Autodesk Inventor part; units mm, degrees
ref_plane "Arbeitsebene1" through (0, 0, -100) normal (0, 0, -1) x (-1, 0, 0)
ref_plane "Arbeitsebene3" through (0, 0, -113.5) normal (0, 0, -1) x (-1, 0, 0)
ref_plane "Arbeitsebene4" through (-9.5, -5.25, -113.5) normal (-1, 0, 0) x (0, 0, 1)
sketch "Skizze1" plane through (0, 0, 0) normal (0, 0, 1) x (1, 0, 0)
  line L0 (-9.5, -10.5) -> (7.5, -10.5)
  line L1 (7.5, -10.5) -> (7.5, 10.5)
  line L2 (7.5, 10.5) -> (-9.5, 10.5)
  line L3 (-14.1, 0) -> (18.1, 0)
  line L4 (0, -21.7) -> (0, 21.7)
  line L5 (-9.5, -10.5) -> (-9.5, -15.5)
  line L6 (-9.5, -15.5) -> (13.5, -15.5)
  line L7 (-9.5, 10.5) -> (-9.5, 15.5)
  line L8 (-9.5, 15.5) -> (13.5, 15.5)
  line L9 (13.5, 15.5) -> (13.5, -15.5)
  point P0 (0, 0)
  dimension "d2" = 21
  dimension "d4" = 7.5
  dimension "d5" = 5
  dimension "d8" = 5
  dimension "d9" = 23
  dimension "d147" = 6
  dimension "d148" = 23
extrude "Tower" add sketch "Skizze1" against normal blind 100 contours L0 L4 L6 L5 | L0 L1 L3 L9 L6 L4 | L1 L2 L4 L8 L9 L3 | L2 L7 L8 L4
ref_plane "Arbeitsebene1" through (0, 0, -100) normal (0, 0, -1) x (-1, 0, 0)
sketch "Skizze6" plane through (-9.5, 15.5, 0) normal (0, 1, 0) x (1, 0, 0)
  line L0 (0, 0) -> (23, 0)
  line L1 (0, 0) -> (0, -10)
  line L2 (0, -10) -> (228, -10)
  line L3 (23, 0) -> (23, 100)
  line L4 (0, -10) -> (246, -10)
  line L5 (246, -10) -> (246, 46)
  line L6 (246, 46) -> (224, 46)
  line L7 (246, 46) -> (268, 46) construction
  line L8 (23, 71.167) -> (23, 0)
  line L9 (0, 0) -> (17, 0)
  line L10 (0, 0) -> (0, -12)
  line L11 (246, -12) -> (246, -10)
  spline S0 degree 4 poles (224, 46) (217.2503, 45.4128) (195.5245, 22.479) (125.572, 22.5752) (22.0276, 45.7385) (23, 71.167) knots 0 0 0 0 0 0.374897 1 1 1 1 1
  line L12 (221.3219, 44.8948) -> (192.3718, 31.261) construction
  arc A0 (195.0075, 33.4464) -> (217.9584, 44.255) centre (166.5411, 123.6635) ccw construction
  line L13 (148.8192, 27.3272) -> (94.421, 32.9509) construction
  arc A1 (99.9704, 33.0497) -> (143.4073, 28.5591) centre (158.3015, 384.9585) ccw construction
  line L14 (0, 0) -> (0, 100)
  point P0 (9.5, 0)
  point P1 (206.8469, 38.0779)
  point P2 (121.6201, 30.1391)
  point P3 (23, 70.1618)
  dimension "d34" = 10
  dimension "d38" = 246
  dimension "d39" = 56
  dimension "d40" = 180
  dimension "d41" = 22
extrude "Gripperbogen" add sketch "Skizze6" against normal blind 31 contours L0 L3 S0 L6 L5 L4 L2 L1
sketch "Skizze9" plane through (-9.5, 15.5, 10) normal (0, 0, 1) x (1, 0, 0)
  line L0 (216, -15.5) -> (246, -15.5)
  line L1 (246, 0) -> (246, -31)
  line L2 (216, -15.5) -> (246, -15.5) construction
  line L3 (246, -15.5) -> (246, -31)
  line L4 (224, 0) -> (224, -31)
  line L5 (246, -9.5) -> (224, -9.5)
  line L6 (224, -9.5) -> (224, -6)
  line L7 (224, -6) -> (246, -6)
  line L8 (246, -6) -> (246, -9.5)
  line L9 (0, 0) -> (246, 0)
  line L10 (0, 0) -> (246, 0)
  line L11 (0, 0) -> (0, -31)
  line L12 (246, -31) -> (0, -31)
  line L13 (246, 0) -> (246, -31)
  line L14 (216, -15.5) -> (146, -31)
  point P0 (9.5, -15.5)
  point P1 (246, -6)
  point P2 (235, -6)
  dimension "d61" = 3.5
  dimension "d150" = 6
  dimension "d151" = 6
  dimension "d152" = 100
  dimension "d153" = 30
extrude "Extrusion8" cut sketch "Skizze9" against normal blind 74.5 contours L0 L4 L12 L14 | L0 L1 L12 L4 | L4 L7 L1 L5
sketch "Skizze10" plane through (-9.5, 15.5, -100) normal (0, 1, 0) x (1, 0, 0)
  line L0 (225.7282, -61.6) -> (255.0049, -61.6)
  line L1 (255.0049, -61.6) -> (255.0049, -102.4)
  line L2 (255.0049, -102.4) -> (225.7282, -102.4)
  line L3 (225.7282, -102.4) -> (225.7282, -61.6)
  line L4 (0, -110) -> (246, -110)
  line L5 (246, -54) -> (224, -54)
  point P0 (9.5, -100)
  dimension "d64" = 7.6
  dimension "d65" = 7.6
extrude "Extrusion9" cut sketch "Skizze10" against normal blind 74.5
sketch "Skizze12" plane through (0, 0, -100) normal (0, 0, -1) x (-1, 0, 0)
  line L0 (-214.5, 9.5) -> (-236.5, 9.5)
  line L1 (-236.5, 15.5) -> (-236.5, 9.5)
  line L2 (9.5, 15.5) -> (-236.5, 15.5)
  line L3 (9.5, 15.5) -> (9.5, -15.5)
  line L4 (-136.5, -15.5) -> (9.5, -15.5)
  line L5 (-136.5, -15.5) -> (-206.5, 0)
  line L6 (-206.5, 0) -> (-236.5, 0)
  line L7 (-236.5, 6) -> (-236.5, 0)
  line L8 (-236.5, 6) -> (-214.5, 6)
  line L9 (-214.5, 6) -> (-214.5, 9.5)
  line L10 (-7.5, 10.5) -> (9.5, 10.5)
  line L11 (9.5, 10.5) -> (9.5, 15.5)
  line L12 (9.5, 15.5) -> (-13.5, 15.5)
  line L13 (-13.5, 15.5) -> (-13.5, -15.5)
  line L14 (-13.5, -15.5) -> (9.5, -15.5)
  line L15 (9.5, -15.5) -> (9.5, -10.5)
  line L16 (9.5, -10.5) -> (-7.5, -10.5)
  line L17 (-7.5, -10.5) -> (-7.5, 10.5)
  line L18 (-13.5, 15.5) -> (-13.5, -15.5)
  line L19 (-13.5, -15.5) -> (9.5, -15.5)
  line L20 (9.5, -15.5) -> (9.5, 15.5)
  line L21 (9.5, 15.5) -> (-13.5, 15.5)
  line L22 (-13.5, 15.5) -> (-13.5, -15.5)
  point P0 (9.5, 25.25)
  point P1 (-13.5, -5.25)
  point P2 (-13.5, 15.5)
extrude "Extrusion10" add sketch "Skizze12" against normal blind 10 contours L2 L3 L10 L17 L16 L4 L13 | L3 L16 L17 L10
ref_plane "Arbeitsebene3" through (0, 0, -113.5) normal (0, 0, -1) x (-1, 0, 0)
ref_plane "Arbeitsebene4" through (-9.5, -5.25, -113.5) normal (-1, 0, 0) x (0, 0, 1)
sketch "Skizze18" plane through (0, 0, -90) normal (0, 0, 1) x (1, 0, 0)
  line L0 (7.5, 10.5) -> (7.5, -10.5)
  line L1 (-9.5, 10.5) -> (7.5, 10.5)
  circle A0 centre (2, 0) radius 2.75
  line L2 (7.5, -10.5) -> (-9.5, -10.5)
  line L3 (-9.5, 10.5) -> (-9.5, -10.5)
  point P0 (0, 0)
  dimension "d132" = 5.5
  dimension "d154" = 0
  dimension "d155" = 11.5
  dimension "d161" = 21
  dimension "d162" = 17
extrude "Extrusion15" cut sketch "Skizze18" against normal through all contours A0
sketch "Skizze19" plane through (-9.5, -15.5, -100) normal (-1, 0, 0) x (0, 0, 1)
  line L0 (0, 0) -> (0, 31)
  line L1 (110, 0) -> (0, 0)
  line L2 (110, 31) -> (110, 0)
  line L3 (0, 31) -> (110, 31)
  line L4 (100, 26) -> (10, 26)
  line L5 (100, 26) -> (100, 5)
  line L6 (100, 5) -> (10, 5)
  line L7 (60, 31) -> (60, 0)
  line L8 (10, 26) -> (10, 5)
  line L9 (10, 26) -> (0, 26)
  line L10 (10, 5) -> (0, 5)
  line L11 (100, 26) -> (110, 26)
  line L12 (10, 26) -> (10, 5)
  point P0 (100, 15.5)
  point P1 (23.5, 25.5)
  point P2 (23.5, 5)
  point P3 (60, 26)
  point P4 (60, 5)
  point P5 (20, 10.25)
  dimension "d113" = 50
extrude "Extrusion16" add sketch "Skizze19" along normal blind 70 contours L11 L4 L7 L3 L2
sketch "Skizze27" plane through (206.3978, 0, 10) normal (0, -1, 0) x (1, 0, 0)
  line L0 (9.8304, -7.6) -> (30.1022, -7.6)
  line L1 (30.1022, 0) -> (30.1022, -7.6)
  line L2 (0.1022, 0) -> (30.1022, 0)
  line L3 (0.1022, 0) -> (0.1022, -52.845)
  line L4 (30.1022, -56) -> (8.1022, -56)
  line L5 (30.1022, -48.4) -> (30.1022, -56)
  line L6 (30.1022, -48.4) -> (9.8304, -48.4)
  line L7 (9.8304, -48.4) -> (9.8304, -7.6)
  circle A0 centre (25.1022, -3.8) radius 1.6
  circle A1 centre (15.1022, -3.8) radius 1.6
  line L8 (30.1022, 0) -> (30.1022, -7.6)
  circle A2 centre (25.1022, -52.2) radius 1.6
  circle A3 centre (15.1022, -52.2) radius 1.6
  point P0 (-206.3978, -10)
  point P1 (30.1022, -3.8)
  point P2 (28.2249, -52.2)
  point P3 (30.1022, -52.2)
  dimension "d120" = 3.2
  dimension "d121" = 5
  dimension "d122" = 3.2
  dimension "d123" = 10
  dimension "d127" = 3.2
  dimension "d129" = 3.2
extrude "Extrusion18" cut sketch "Skizze27" against normal blind 20
sketch "Skizze15" plane through (-9.5, -15.5, -100) normal (0, -1, 0) x (1, 0, 0)
  line L0 (23, 0) -> (0, 0)
  line L1 (23, 29.8382) -> (23, 0)
  circle A0 centre (9.5, 48) radius 2.25
  circle A1 centre (9.5, 88) radius 2.25
  line L2 (146, 110) -> (0, 110)
  line L3 (0, 110) -> (0, 0)
  line L4 (146, 71.4914) -> (146, 110)
  point P0 (9.5, 100)
  dimension "d138" = 4.5
  dimension "d142" = 4.5
  dimension "d143" = 40
  dimension "d156" = 22
  dimension "d157" = 9.5
extrude "Extrusion13" cut sketch "Skizze15" against normal blind 100
sketch "Skizze32" plane through (-9.5, -15.5, 10) normal (0, 0, 1) x (1, 0, 0)
  circle A0 centre (11.5, 15.5) radius 2.75
  line L0 (0, 0) -> (0, 31)
  line L1 (0, 31) -> (23, 31)
  line L2 (23, 31) -> (23, 0)
  line L3 (23, 0) -> (0, 0)
  circle A1 centre (11.5, 15.5) radius 1.75
  point P0 (9.5, 15.5)
  dimension "d158" = 3.5
extrude "Extrusion20" cut sketch "Skizze32" against normal blind 10 contours A1
sketch "Skizze34" plane through (0, 0, -100) normal (0, 0, -1) x (-1, 0, 0)
  circle A0 centre (-2, 0) radius 2.75
  line L0 (9.5, -15.5) -> (9.5, 15.5)
  line L1 (9.5, 15.5) -> (-13.5, 15.5)
  line L2 (-13.5, 15.5) -> (-13.5, -15.5)
  line L3 (-13.5, -15.5) -> (9.5, -15.5)
  point P0 (0, 0)
  dimension "d171" = 23
  dimension "d172" = 31
  dimension "d173" = 15.5
  dimension "d174" = 11.5
  dimension "d175" = 5.5
sketch "Skizze35" plane through (13.5, -15.5, -100) normal (1, 0, 0) x (0, 0, -1)
  line L0 (-29.8382, 31) -> (0, 31)
  line L1 (-29.8382, 0) -> (0, 0)
  line L2 (0, 31) -> (0, 0)
  line L3 (-29.8382, 31) -> (0, 31)
  line L4 (-29.8382, 31) -> (-29.8382, 0)
  line L5 (-29.8382, 0) -> (0, 0)
  line L6 (0, 31) -> (0, 0)
  line L7 (0, 0) -> (-5, 0)
  line L8 (-5, 0) -> (-5, 31)
  line L9 (-5, 31) -> (0, 31)
  line L10 (0, 31) -> (0, 0)
  point P0 (-100, 15.5)
  point P1 (-5, 31)
  point P2 (-5, 0)
  dimension "d176" = 5
extrude "Extrusion22" add sketch "Skizze35" along normal blind 10 contours L0 L2 L1 L8
sketch "Skizze36" plane through (23.5, -15.5, -100) normal (1, 0, 0) x (0, 0, -1)
  line L0 (-5, 0) -> (0, 0)
  line L1 (0, 0) -> (0, 31)
  line L2 (0, 31) -> (-5, 31)
  line L3 (-5, 31) -> (-5, 0)
  arc A0 (-9.879, -89.9986) -> (-9.879, 121.0014) centre (-1120.404, 15.5014) ccw
  line L4 (-5, 15.5) -> (0, 15.5)
  arc A1 (-4.9014, -90.4715) -> (-4.9014, 121.4742) centre (-1120.404, 15.5014) ccw
  line L5 (-5, 15.5) -> (0, 15.5)
  line L6 (-14.7679, -34.5) -> (17.3967, -34.5)
  line L7 (-14.7679, 65.5) -> (14.0644, 65.5)
  point P0 (-100, 15.5)
  point P1 (-0.9951, 65.5)
  point P2 (-6.0001, 65.5)
  point P3 (-4.9867, 31)
  point P4 (-4.9867, 0)
  point P5 (-6.0002, -34.5)
  point P6 (-0.9952, -34.5)
  dimension "d181" = 5
  dimension "d182" = 100
extrude "Extrusion23" add sketch "Skizze36" along normal blind 10
sketch "Skizze40" plane through (206.5, 0, 10) normal (0, -1, 0) x (1, 0, 0)
  circle A0 centre (15, -52.2) radius 1.6
  circle A1 centre (15, -3.8) radius 1.6
  circle A2 centre (25, -52.2) radius 1.6
  circle A3 centre (25, -3.8) radius 1.6
  circle A4 centre (15, -3.8) radius 2.1
  circle A5 centre (25, -3.8) radius 2.1
  circle A6 centre (15, -52.2) radius 2.1
  circle A7 centre (25, -52.2) radius 2.1
  point P0 (-206.5, -10)
  dimension "d198" = 4.2
  dimension "d199" = 4.2
  dimension "d200" = 4.2
  dimension "d201" = 4.2
extrude "Extrusion27" cut sketch "Skizze40" against normal blind 6 contours A0 | A1 | A2 | A3 | A4 | A5 | A6 | A7
sketch "Skizze41" plane through (-9.5, 10.5, 0) normal (0, -1, 0) x (1, 0, 0)
  line L0 (0, 10) -> (-70, 10)
  line L1 (-70, -40) -> (-70, 10)
  line L2 (0, -40) -> (-70, -40)
  line L3 (-70, 10) -> (-58, 10)
  line L4 (-58, 10) -> (-58, 6)
  line L5 (-58, 6) -> (-70, 6)
  line L6 (-70, 6) -> (-70, 10)
  line L7 (-70, -40) -> (-58, -40)
  line L8 (-58, -40) -> (-58, -36)
  line L9 (-58, -36) -> (-70, -36)
  line L10 (-70, -36) -> (-70, -40)
  line L11 (-70, -25) -> (-70, -21)
  line L12 (-70, -9) -> (-70, -5)
  line L13 (-70, -15) -> (0, -15)
  line L14 (0, 10) -> (0, -100)
  line L15 (-70, -13) -> (-58, -13)
  line L16 (-58, -13) -> (-58, -17)
  line L17 (-58, -17) -> (-70, -17)
  line L18 (-70, -17) -> (-70, -13)
  point P0 (9.5, 0)
  point P1 (-70, -36)
  point P2 (-70, 6)
  point P3 (-58, 8)
  point P4 (-58, -15)
  point P5 (-58, -38)
  point P6 (-70, -17)
  dimension "d204" = 12
  dimension "d205" = 4
  dimension "d207" = 4
  dimension "d222" = 4
extrude "Extrusion28" add sketch "Skizze41" along normal blind 9 contours L4 L5 L1 L0 | L16 L17 L1 L13 | L13 L1 L15 L16 | L2 L1 L9 L8
sketch "Skizze42" plane through (-9.5, -15.5, 10) normal (0, 0, 1) x (1, 0, 0)
  line L0 (-58, 17) -> (-70, 17)
  line L1 (-70, 26) -> (-58, 26)
  line L2 (-58, 26) -> (-70, 26)
  line L3 (-64, 26) -> (-64, 17)
  line L4 (-61, 26) -> (-67, 26)
  line L5 (-70, 31) -> (-70, 17)
  line L6 (-58, 26) -> (-58, 17)
  circle A0 centre (-64, 23) radius 3
  arc A1 (-70, 23) -> (-58, 23) centre (-64, 23) ccw
  point P0 (9.5, 15.5)
  point P1 (0, 17)
  dimension "d220" = 6
  dimension "d221" = 3
extrude "Extrusion29" cut sketch "Skizze42" against normal blind 100 contours L0 A1 L6 | L0 L5 A1 | A0 L3 | L3 A0
properties part number "Korpus"
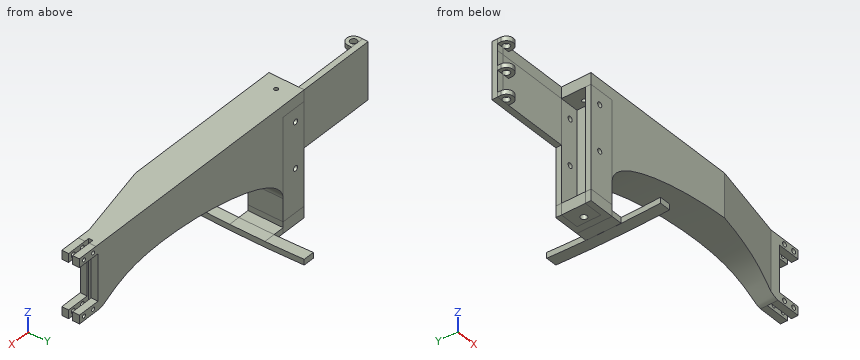
Can you work these out from the model? Positions are in its coordinate system, mm. Round coordinates to 2 decimals unless told otherwise and drop trailing zeros. Loops run counter-clockwise (first coordinate to the right, second up) from the corner with the lowest first, then second, coordinate; pieces in that order, holes last.
Item 1: Please list where these lines run through material, in increasing order: L1, parallel to X at y = 7.5, z = -16; L2, parallel to Z at x = 0, y = 13.9; L3, parallel to Z at x = 221, y = 2.
Item 2: Suppose I cut it at B-B, the plane y = -24.5. Write out the boundary of the cut face in (x, z).
Item 3: Will these pins go through, and if not, where does the flat tip stop? pin 1 Ø6.5 at (y, z) = (-4, -43) entering from -X; pin 2 Ø4 at (x, z) = (58.5, -22) entering from +Y; pin 3 Ø1.8 at (x, z) = (-77, -6) entering from -Y.
Item 4: Suppose I cut it at A-A, the plane x = 10.5. Write out the boundary of the cut face in (y, z), then the cut area to 3 significant figures.
Reported:
1. L1: x = -79.5 to -76.5, -70.5 to -67.5, 7.5 to 214.5
1. L2: z = -100 to -54.25, -49.75 to -14.25, -9.75 to 10
1. L3: z = -46 to -44.24, -40.16 to -38.4, 2.4 to 4.16, 8.24 to 10
2. outline: (23.5, -99.85) - (33.5, -99.85) - (33.5, -94.85) - (23.5, -94.85) - close
3. pin 1: stops at x = 7.5
3. pin 2: stops at y = 15.5
3. pin 3: stops at y = 10.5
4. outline: (-15.5, -100) - (15.5, -100) - (15.5, 10) - (-15.5, 10) - close
4. area: 3,410 mm2
